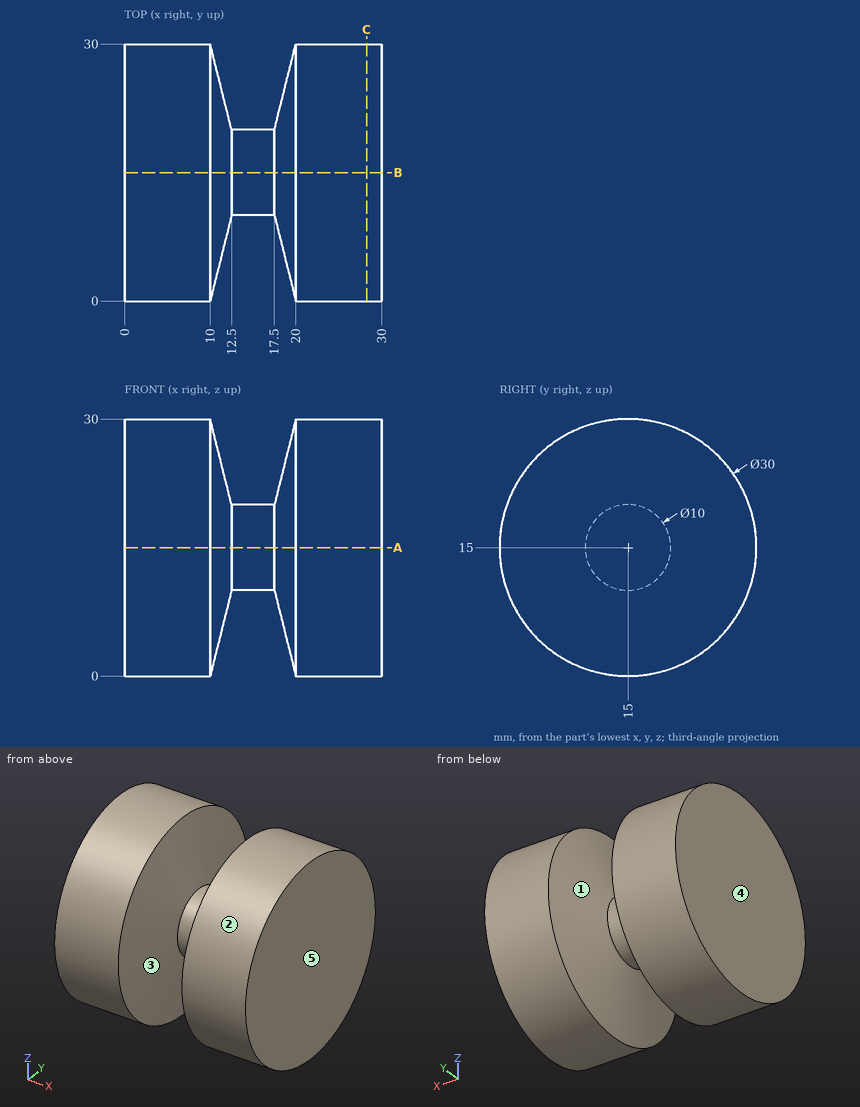
Drawing for the job (mm, zero at the part's lowest x, y, z). A direction names the side the tool comes from. Round coordinates to 2 decimals unless told otherwise and drop trailing zeros. Order: outer loops, then holes, each group sorted by start corner. A loop starts at its lowest first (then second) coordinate and runs counter-clockwise, first axis right, second up.
Item 1: Mould opens along X. For the marked faces 3, 4 and 5 say: pulls with the +X half, pulls with the -X half, needs draft (parallel to the pull), parting line crosses it, or undercut.
Item 2: Pin check, flat tips, straight feed: pin 1 (5 mm diameter, centred on y = 10.5, z = 14, fed in from -X); pin 2 (2 mm diameter, centred on x = 23.5, y = 20.5, fed in from -Z). Stop position of each tip, or through.
Item 3: Probe line 1 along X through (y, z) = (12.5, 21) (3 decimals); line 2 along X through (y, z) = (23, 20); line 3 along Z through (x, y) = (4.5, 23.25). List the from-to ranges inside material, lowest first.
Item 4: Saw through at A-A on z = 15. Write the cut outline in (x, y).
Item 5: Tool access for the marked faces 1 and 2: list every direction of +Z, -Z, +X, -X, +Y, -Y with a clear straight run to the whole face (end or side of a thin tool).
Item 6: Saw through at C-C on x = 28.25. Write the cut outline in (y, z), then the cut area to 3 significant figures.
Reported:
1. face 3: undercut
1. face 4: pulls with the -X half
1. face 5: pulls with the +X half
2. pin 1: stops at x = 0
2. pin 2: stops at z = 0.69
3. line 1: x = 0 to 12.125, 17.875 to 30
3. line 2: x = 0 to 11.39, 18.61 to 30
3. line 3: z = 2.47 to 27.53
4. outline: (0, 0) - (10, 0) - (12.5, 10) - (17.5, 10) - (20, 0) - (30, 0) - (30, 30) - (20, 30) - (17.5, 20) - (12.5, 20) - (10, 30) - (0, 30) - close
5. face 1: none
5. face 2: +X, -X
6. outline: circle Ø30 at (15, 15)
6. area: 707 mm2
